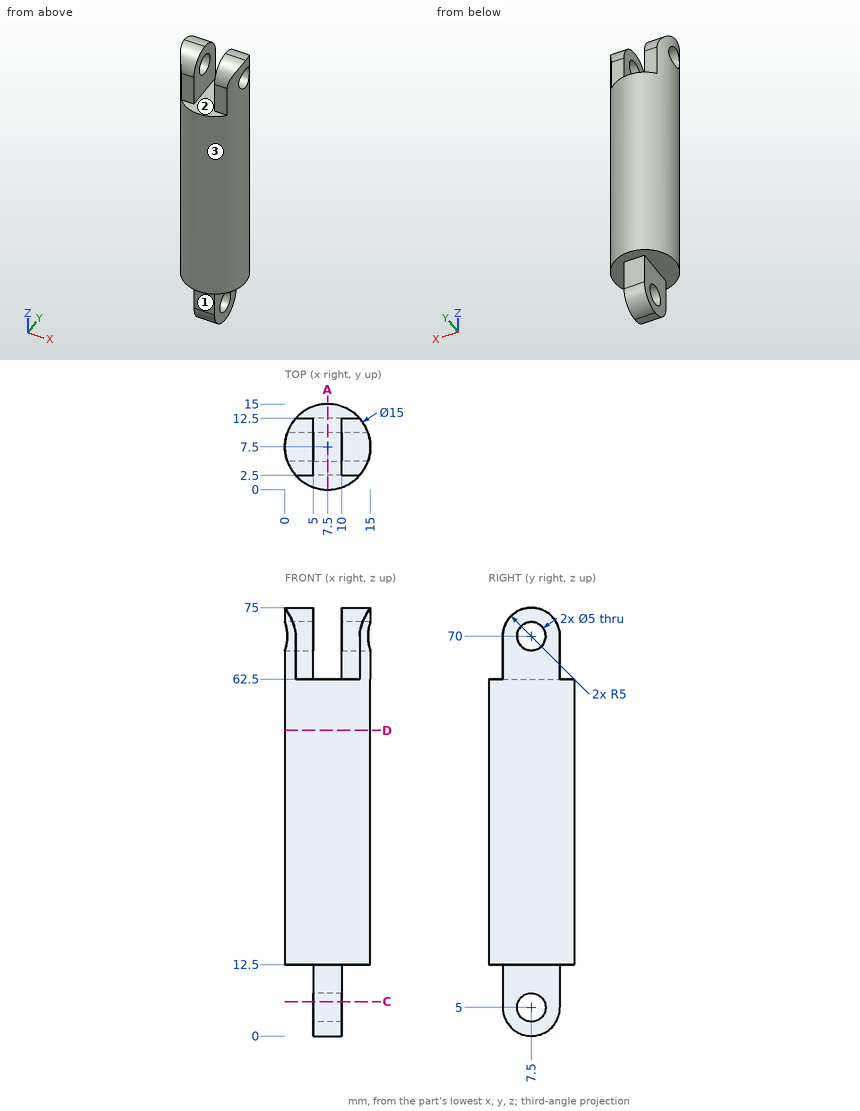
Check sheet for the drawn part. Datum: minimum x, y, z corner. Units: mm. Coordinates: 2 decimals unless noted, no trailing zeros. Order: outer loops, then holes, each group sorted by start corner. A loop starts at its lowest first (then second) coordinate and runs counter-clockwise, first axis right, second up. Notation, with made-up numbers: M 55.25,87.5 L 62.25,87.5 A23 cw 62.25,98.5 Z; hole C -29.75,37 d2. An arc over 180 degrees is marked long. One line per question, with ' | ' between items. Start each with the question number.
Item 1: Gauge pin test, flat ends, axial feed: pin 1 (0.9 mm diameter, centred on x = 11, z = 66.5, fed in from -Y); pin 2 (4 mm diameter, centred on x = 12, z = 21, fed in from -Y); pin 3 (6.5 mm diameter, centred on y = 7.5, z = 5, fed in from -X). Record the tip position at first contact, or that the pin passes through.
Item 2: Cross-section at A-A on x = 7.5. Enter the section's corners in (y, z), then the cut area to 3 significant figures.
Item 3: Cross-section at D-D on z = 53.5. Enter the section's corners in (x, y).
Item 4: Draft check along X on the marked faces 1, 2 and 3. Enter one of: pulls with the +X half, pulls with the -X half, needs draft (parallel to the pull), parting line crosses it, or undercut.
Item 5: Material ranges on L1, parallel to Y at x = 11.5, z = 70; L2, parallel to Z at x = 7, y = 2; L3, parallel to Y at x = 1.75, z = 70, recorded low to high. Write a range as [from, to].
Item 6: Cross-section at C-C on z = 6. Enter the section's corners in (x, y), then the cut area to 3 significant figures.
Findings:
1) pin 1: stops at y = 2.5 | pin 2: stops at y = 0.43 | pin 3: stops at x = 5
2) outline: M 0,12.5 L 2.5,12.5 L 2.5,5 A5 ccw 12.5,5 L 12.5,12.5 L 15,12.5 L 15,62.5 L 0,62.5 Z; hole C 7.5,5 d5 | area: 845 mm²
3) outline: C 7.5,7.5 d15
4) face 1: needs draft | face 2: undercut | face 3: parting line crosses it
5) L1: y = [2.5, 5], [10, 12.5] | L2: z = [12.5, 62.5] | L3: y = [2.68, 5], [10, 12.32]
6) outline: M 5,2.5 L 10,2.5 L 10,5.21 L 5,5.21 Z; M 5,9.79 L 10,9.79 L 10,12.5 L 5,12.5 Z | area: 27.1 mm²
